For this review, take the finished solid that the model builds, in its own axes (mm). A direction names the side the tool comes from. Round coordinates to 2 decimals unless told otherwise and drop trailing zeros. Order: outer loops, then holes, each group sorted by start corner. A loop starts at its lowest first (then second) coordinate and runs counter-clockwise, first axis right, second up.
Autodesk Inventor part; units mm, degrees
ref_plane "YZ Plane" through (0, 0, 0) normal (1, 0, 0) x (0, 1, 0)
ref_plane "XZ Plane" through (0, 0, 0) normal (0, 1, 0) x (-1, 0, 0)
ref_plane "XY Plane" through (0, 0, 0) normal (0, 0, 1) x (1, 0, 0)
sketch "Sketch1" plane through (0, 0, 0) normal (1, 0, 0) x (0, 1, 0)
  line L0 (0, 0) -> (120, 0)
  line L1 (120, 0) -> (120, -95)
  line L2 (120, -95) -> (0, -95)
  line L3 (0, -95) -> (0, 0)
  dimension "d0" = 120
  dimension "d1" = 95
extrude "Extrusion1" add sketch "Sketch1" along normal blind 6
sketch "Sketch2" plane through (6, 0, 0) normal (1, 0, 0) x (0, 0, -1)
  line L0 (0, 120) -> (0, 0)
  line L1 (0, 0) -> (95, 0)
  line L2 (95, 0) -> (95, 120)
  line L3 (95, 120) -> (0, 120)
  line L4 (0, 120) -> (0, 0)
  line L5 (0, 15) -> (5.875, 15)
  line L6 (5.875, 15) -> (5.875, 45)
  line L7 (5.875, 45) -> (0, 45)
  line L8 (0, 45) -> (0, 15)
  line L9 (0, 75) -> (5.875, 75)
  line L10 (5.875, 75) -> (5.875, 105)
  line L11 (5.875, 105) -> (0, 105)
  line L12 (0, 105) -> (0, 75)
  line L13 (95, 15) -> (89.125, 15)
  line L14 (89.125, 15) -> (89.125, 45)
  line L15 (89.125, 45) -> (95, 45)
  line L16 (95, 45) -> (95, 15)
  line L17 (95, 75) -> (89.125, 75)
  line L18 (89.125, 75) -> (89.125, 105)
  line L19 (89.125, 105) -> (95, 105)
  line L20 (95, 105) -> (95, 75)
  line L21 (-12.0657, 60) -> (104.2665, 60)
  line L22 (95, 120) -> (0, 120)
  dimension "d5" = 5.875
  dimension "d6" = 5.875
  dimension "d8" = 30
  dimension "d9" = 30
  dimension "d22" = 60
  dimension "d23" = 15
  dimension "d24" = 15
extrude "Extrusion2" cut sketch "Sketch2" against normal up to next contours L11 L10 L9 L0 | L2 L17 L18 L19 | L7 L6 L5 L0 | L2 L13 L14 L15
sketch "Sketch3" plane through (6, 0, 0) normal (1, 0, 0) x (0, 0, -1)
  circle A0 centre (75, 10) radius 2.5
  circle A1 centre (75, 110) radius 2.5
  line L0 (95, 105) -> (95, 120)
  line L1 (95, 120) -> (0, 120)
  line L2 (95, 0) -> (95, 15)
  line L3 (0, 0) -> (95, 0)
  dimension "d13" = 20
  dimension "d14" = 10
  dimension "d15" = 5
  dimension "d17" = 10
  dimension "d18" = 20
  dimension "d19" = 5
extrude "Extrusion3" cut sketch "Sketch3" against normal up to next
properties part number "Side"
Q1. Clearance check with flat-ended pins moving along their axes: pin 1 (1.5 mm diameter, centred on x = 3, y = 17, fed in from +Z) (3 decimals); pin 2 (1 mm diameter, centred on x = 1.5, y = 39, fed in from -Z) (3 decimals). State where each tip first meets the part, or that it passes through.
Q2. Take a section at C-C, the plane x = 4.15. State the section outline as (y, z) points (3 decimals), plus the area to 3 significant figures.
Q3. Wall thickness on line 1 (Y direction, x = 4.05, z = -75); line 2 (Z direction, x = 1.7, y = 84) (3 decimals); line 3 (Z direction, x = 0.45, y = 11): over which ranges is each line inside the solid? List them lowest first.
Q4. Take a section at B-B, the plane z = -75. State the section outline as (x, y) points.
Q5. Take a section at A-A, the plane y = 110. State the section outline as (x, z) points, plus the area to 3 significant figures.
Q6. Mouldability with a two-part tool opening along Y and no side actions: class faces 1 (the face through (6, 59, -47)), 2 (the face through (3, 0, -48)), 3 (the face through (3, 90, -5.875)) as +Y half, -Y half, draft (parallel to the pull), parting line (faces both ways), or undercut.
Q7. Tool access review of faces 4 (the face through (3, 8.5, -73)), 5 (the face through (3, 45, -3)), 6 (the face through (3, 30, -89.125)): name each direction out of +Z, -Z, +X, -X, +Y, -Y from which nothing blocks a thin tool from reaching the whole face with its end or side.
Working result:
1. pin 1: stops at z = -5.875
1. pin 2: stops at z = -89.125
2. outline: (0, -95) - (15, -95) - (15, -89.125) - (45, -89.125) - (45, -95) - (75, -95) - (75, -89.125) - (105, -89.125) - (105, -95) - (120, -95) - (120, 0) - (105, 0) - (105, -5.875) - (75, -5.875) - (75, 0) - (45, 0) - (45, -5.875) - (15, -5.875) - (15, 0) - (0, 0) - close; hole circle Ø5 at (10, -75); hole circle Ø5 at (110, -75)
2. area: 10,700 mm2
3. line 1: y = 0 to 7.5, 12.5 to 107.5, 112.5 to 120
3. line 2: z = -89.125 to -5.875
3. line 3: z = -95 to -77.29, -72.71 to 0
4. outline: (0, 0) - (6, 0) - (6, 7.5) - (0, 7.5) - close; (0, 12.5) - (6, 12.5) - (6, 107.5) - (0, 107.5) - close; (0, 112.5) - (6, 112.5) - (6, 120) - (0, 120) - close
5. outline: (0, -95) - (6, -95) - (6, -77.5) - (0, -77.5) - close; (0, -72.5) - (6, -72.5) - (6, 0) - (0, 0) - close
5. area: 540 mm2
6. face 1: draft
6. face 2: -Y half
6. face 3: undercut
7. face 4: +X, -X
7. face 5: +Z, +X, -X
7. face 6: -Z, +X, -X
